Geometry check sheet. Reference: drawing and pictorial views, mm from the part's lowest x, y, z. Give positions to 0.01 mm unless a question says otherwise; leave off trailing zeros. Write each loop counter-clockwise with the first axis right and the second up, starting at its lowest first coordinate (ties: lowest second). Pieces come first, ordered by that corner, then holes. Notation, with made-up numbers: (-8.5, -18) - (31.5, -18) arc R31 ccw to (31.5, 11) - close; hole circle Ø4 at (-29, 89.25). An arc over 180 degrees is marked (long way). Put each result on its own line as item: value.
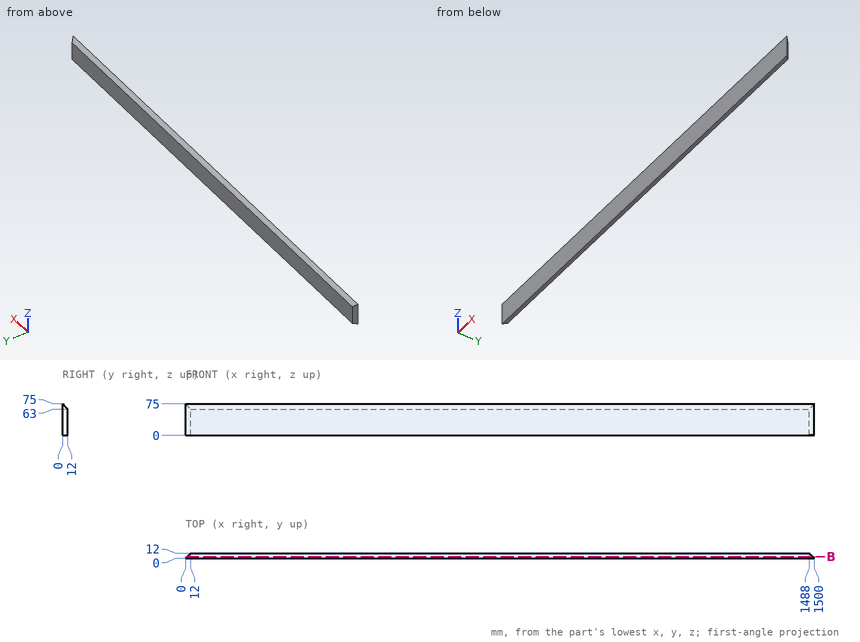
Q1. Section check B-B, the plane y = 4.5. Record the cut outline in (x, z), plus the area to 3 significant figures.
Answers follow:
outline: (4.5, 0) - (1495.5, 0) - (1495.5, 70.5) - (4.5, 70.5) - close
area: 105,000 mm2
Q2. Scan lines: line 1 along Z through (x, y) = (625, 2); line 2 along X through (y, z) = (4.75, 23); line 3 along Z through (x, y) = (989, 7). Record each from-to range of solid material in increasing order.
Answers follow:
line 1: z = 0 to 73
line 2: x = 4.75 to 1495.25
line 3: z = 0 to 68
Q3. Go/stop test with flat-tipped pins: pin 1 Ø3 at (x, y) = (1308, 9.5) entering from +Z; pin 2 Ø1.5 at (x, y) = (957, 8.5) entering from +Z; pin 3 Ø2 at (y, z) = (6, 12) entering from -X. Record where each tip stops, or that it passes through.
Answers follow:
pin 1: stops at z = 67
pin 2: stops at z = 67.25
pin 3: stops at x = 5
